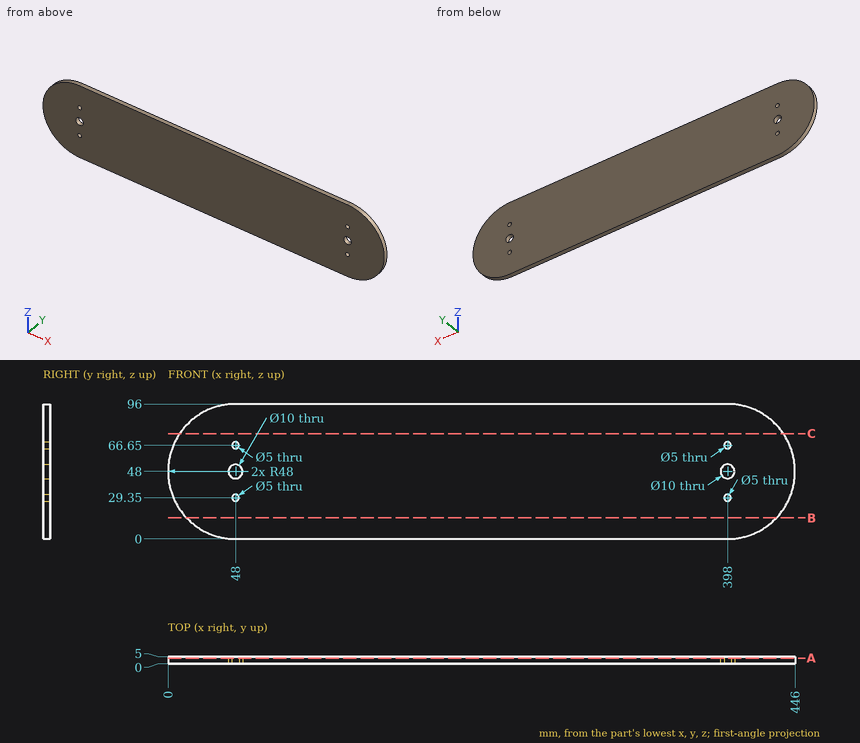
Can you work these out from the drawing? Everything is in mm from the part's minimum corner. Coordinates: 2 decimals unless noted, no trailing zeros. Loops run counter-clockwise (first coordinate to the right, second up) from the corner with the lowest first, then second, coordinate; pieces in that order, holes last. Notation, with made-up numbers: (-0.5, 68) - (11.5, 68) arc R18 cw to (11.5, 73) - close; hole circle Ø2 at (54, 28.5). An arc over 180 degrees is marked (long way). Put each result on its own line as item: value. Start each with the question number.
Item 1: Suppose I cut it at C-C (z = 75). Please give me the cut outline in (x, y), and give its area (3 significant figures).
Item 2: For pin 1 (1 mm diameter, centred on x = 190, y = 3, fed in from -Z); pin 2 (8 mm diameter, centred on x = 398, z = 48, fed in from -Y); pin 3 (1.5 mm diameter, centred on y = 1, z = 55, fed in from -X), each with a flat end and sliding along its axis, tell me the tip position at first contact or that it passes through.
Item 3: Suppose I cut it at A-A (y = 4.15). Please give me the cut outline in (x, z), and give its area (3 significant figures).
Item 4: Suppose I cut it at B-B (z = 15). Please give me the cut outline in (x, y).
Item 5: If I drill on line 1 along Z through (x, y) = (48, 3.75); line 2 along X through (y, z) = (1.95, 48); line 3 along X through (y, z) = (3.05, 66.65), over which ranges is the centre line in solid material (lowest first)?
Here are the results:
1. outline: (8.31, 0) - (437.69, 0) - (437.69, 5) - (8.31, 5) - close
1. area: 2,150 mm²
2. pin 1: z = 0
2. pin 2: through
2. pin 3: x = 0.41
3. outline: (48, 0) - (398, 0) arc R48 ccw to (398, 96) - (48, 96) arc R48 ccw to start; hole circle Ø10 at (48, 48); hole circle Ø5 at (48, 29.35); hole circle Ø5 at (48, 66.65); hole circle Ø10 at (398, 48); hole circle Ø5 at (398, 29.35); hole circle Ø5 at (398, 66.65)
3. area: 40,600 mm²
4. outline: (13.14, 0) - (432.86, 0) - (432.86, 5) - (13.14, 5) - close
5. line 1: 0 to 26.85, 31.85 to 43, 53 to 64.15, 69.15 to 96
5. line 2: 0 to 43, 53 to 393, 403 to 446
5. line 3: 3.77 to 45.5, 50.5 to 395.5, 400.5 to 442.23
